```python
from build123d import *

# Parameters (mm, degrees)
BASE_SKETCH_R            = 0.625
BASE_EXTRUDE_DEPTH       = 1.5
CIRCLE_SKETCH_R          = 3.5
CIRCLE_SKETCH_R_2        = 2.5
CIRCLE_EXTRUDE_DEPTH     = 2.5
SCREW_CIRCLE1_SKETCH_R   = 2.5
SCREW_CIRCLE_1_CUT_DEPTH = 0.6
SCREW_CIRCLE2_SKETCH_R   = 1
SCREW_CIRCLE_CUT_DEPTH   = 77.422014171


with BuildPart() as part:
    # Base Sketch → Base Extrude (new body)
    with BuildSketch(Plane.ZY.offset(4)):
        with BuildLine():
            Line((-71.399880191, 12.177847643), (-41.820115259, 8.471741587))
            ThreePointArc((-41.820115259, 8.471741587), (-40.765509681, 7.276309847), (-41.821002543, 6.081661451))
            Line((-41.821002543, 6.081661451), (-71.732639675, 5.206497125))
            ThreePointArc((-71.732639675, 5.206497125), (-75.331019627, 8.871873504), (-71.399880191, 12.177847643))
        make_face()
        with Locations((-45.965270944, 7.46783075)):
            Circle(BASE_SKETCH_R, mode=Mode.SUBTRACT)
        with Locations((-48.961846252, 7.611136109)):
            Circle(BASE_SKETCH_R, mode=Mode.SUBTRACT)
        with Locations((-51.958421559, 7.754441469)):
            Circle(BASE_SKETCH_R, mode=Mode.SUBTRACT)
        with Locations((-42.968695636, 7.32452539)):
            Circle(BASE_SKETCH_R, mode=Mode.SUBTRACT)
    extrude(amount=-BASE_EXTRUDE_DEPTH)

    # Circle Sketch → Circle Extrude (add)
    with BuildSketch(Plane(origin=(-2.5, 0, 0), x_dir=(0, 0, -1), z_dir=(1, 0, 0))):
        with Locations(Location((71.835, 8.705, 0), (0, 0, 97.141485201))):
            Circle(CIRCLE_SKETCH_R)
        with Locations((71.835, 8.705)):
            Circle(CIRCLE_SKETCH_R_2, mode=Mode.SUBTRACT)
    extrude(amount=CIRCLE_EXTRUDE_DEPTH)

    # Screw Circle1 Sketch → Screw Circle 1 Cut (cut)
    with BuildSketch(Plane.ZY.offset(4)):
        with Locations(Location((-71.835, 8.705, 0), (0, 0, 180))):
            Circle(SCREW_CIRCLE1_SKETCH_R)
    extrude(amount=-SCREW_CIRCLE_1_CUT_DEPTH, mode=Mode.SUBTRACT)

    # Screw Circle2 Sketch → Screw Circle Cut (cut, through all)
    with BuildSketch(Plane.ZY.offset(4)):
        with Locations((-71.835, 8.705)):
            Circle(SCREW_CIRCLE2_SKETCH_R)
    extrude(amount=-SCREW_CIRCLE_CUT_DEPTH, mode=Mode.SUBTRACT)


solid = part.part
```
Work out the finished part from the listing and answer in its coordinate system (mm). A direction names the side the tool comes from. Round coordinates to 2 decimals unless told otherwise and drop trailing zeros. Loops run counter-clockwise (first coordinate to the right, second up) from the corner with the lowest first, then second, coordinate; pieces in that order, holes last. Notation, with made-up numbers: (1, 78.5) -> (11, 78.5) arc R12 ccw to (11, 94.5) -> close; hole circle Ø2 at (78, 31.25). An arc over 180 degrees is marked (long way). Write each question's results on one line, items separated by ' | '. Start each with the question number.
1. Given pin 1 Ø4 at (y, z) = (8.705, -71.835) entering from -X; pin 2 Ø1.1 at (y, z) = (7.75, -51.96) entering from +X; pin 3 Ø2 at (x, z) = (-0.5, -70) entering from -Y; pin 4 Ø2.5 at (y, z) = (8.705, -71.835) entering from +X, each flat-ended and moving along its own axis, determine where each tip first touches the part or whether it passes through.
2. Section B-B (z = -46) is taken. Determine the outline of the cut face in (x, y), plus the area to 3 significant figures.
3. Section C-C (x = -0.6) is taken. Determine the outline of the cut face in (y, z) (3 decimals), plus the area to 3 significant figures.
4. A tool of negligible diameter and unlimited length cuts with its end or side. For faces 4 (the face through (-3.4, 10, -72)), 5 (the face through (-2.5, 9, -73)), 6 (the face through (-3.26, 7.352, -43.593)), from which of +Z, -Z, +X, -X, +Y, -Y can it reach the whole face along a straight path? Write none if from no direction.
5. For a pull along Z with two mould halves and no side action, classify faces 1 (the face through (-3.26, 10.35, -56.82)), 2 (the face through (-1.27, 9.46, -74.22)), 3 (the face through (-4, 8, -62)) as +Z half, -Z half, draft (parallel to the pull), parting line (faces both ways), or undercut.
6. Find the intervals of material crossed by probe 1 along X at (y, z) = (9.75, -59.5); probe 2 along Z at (x, y) = (-0.5, 11); probe 3 along Z at (x, y) = (-1.5, 8.75), in increasing order. Write a range as from..to.
7. Section A-A (y = 9.25) is taken. Determine the outline of the cut face in (x, z), plus the area to 3 significant figures.
8. Section D-D (y = 11.5) is taken. Determine the outline of the cut face in (x, z).
Evaluation:
1) pin 1: stops at x = -3.4 | pin 2: passes through | pin 3: stops at y = 5.31 | pin 4: stops at x = -2.5
2) outline: (-4, 5.96) -> (-2.5, 5.96) -> (-2.5, 6.84) -> (-4, 6.84) -> close; (-4, 8.09) -> (-2.5, 8.09) -> (-2.5, 9) -> (-4, 9) -> close | area: 2.68 mm2
3) outline: circle Ø7 at (8.705, -71.835); hole circle Ø5 at (8.705, -71.835) | area: 18.8 mm2
4) face 4: -X | face 5: +X | face 6: +X, -X
5) face 1: +Z half | face 2: undercut | face 3: draft
6) probe 1: x = -4..-2.5 | probe 2: z = -74.48..-72.83, -70.84..-69.19 | probe 3: z = -75.33..-74.33, -69.34..-68.34
7) outline: (-4, -75.29) -> (0, -75.29) -> (0, -74.27) -> (-2.5, -74.27) -> (-2.5, -72.67) -> (-3.4, -72.67) -> (-3.4, -74.27) -> (-4, -74.27) -> close; (-4, -69.4) -> (-3.4, -69.4) -> (-3.4, -71) -> (-2.5, -71) -> (-2.5, -69.4) -> (0, -69.4) -> (0, -68.38) -> (-2.5, -68.38) -> (-2.5, -48.03) -> (-4, -48.03) -> close | area: 41.5 mm2
8) outline: (-4, -73.94) -> (0, -73.94) -> (0, -69.73) -> (-2.5, -69.73) -> (-2.5, -65.99) -> (-4, -65.99) -> close
